Geometry: final body of the model. Coordinates: model frame, mm. A direction names the side the tool comes from. Give positions to 0.01 mm unless a question says otherwise; leave off trailing zeros. Loops run counter-clockwise (first coordinate to the right, second up) from the corner with the lowest first, then second, coordinate; pieces in that order, holes last.
from build123d import *

# Parameters (mm, degrees)
BOSS_EXTRUDE1_DEPTH      = 4.5
BOSS_EXTRUDE1_DEPTH_BACK = 4.5
SKETCH2_R                = 6.25
CUT_EXTRUDE1_DEPTH       = 2.7
CUT_EXTRUDE1_DEPTH_BACK  = 2.7
SKETCH3_R                = 2
CUT_EXTRUDE3_DEPTH       = 18
CHAMFER1_SIZE            = 2


with BuildPart() as part:
    # Sketch1 → Boss-Extrude1 (new body, two sides)
    with BuildSketch(Plane(origin=(0, 0, 0), x_dir=(0, 0, -1), z_dir=(1, 0, 0))) as boss_extrude1_sk:
        with BuildLine():
            Line((5, 8.5), (17.5, 8.5))
            Line((17.5, 8.5), (17.5, -8.5))
            Line((17.5, -8.5), (-17.5, -8.5))
            Line((-17.5, -8.5), (-17.5, 8.5))
            Line((-17.5, 8.5), (-5, 8.5))
            ThreePointArc((-5, 8.5), (0, 3.5), (5, 8.5))
        make_face()
    extrude(amount=BOSS_EXTRUDE1_DEPTH)
    extrude(boss_extrude1_sk.sketch, amount=-BOSS_EXTRUDE1_DEPTH_BACK)

    # Sketch2 → Cut-Extrude1 (cut, two sides)
    with BuildSketch(Plane(origin=(0, 0, 0), x_dir=(0, 0, -1), z_dir=(1, 0, 0))) as cut_extrude1_sk:
        with Locations((0, 8.5)):
            Circle(SKETCH2_R)
    extrude(amount=CUT_EXTRUDE1_DEPTH, mode=Mode.SUBTRACT)
    extrude(cut_extrude1_sk.sketch, amount=-CUT_EXTRUDE1_DEPTH_BACK, mode=Mode.SUBTRACT)

    # Sketch3 → Cut-Extrude3 (cut, through all)
    with BuildSketch(Plane(origin=(0, 8.5, 0), x_dir=(1, 0, 0), z_dir=(0, 1, 0))):
        with Locations((0, 12.5)):
            Circle(SKETCH3_R)
        with Locations((0, -12.5)):
            Circle(SKETCH3_R)
    extrude(amount=-CUT_EXTRUDE3_DEPTH, mode=Mode.SUBTRACT)

    # Chamfer1
    chamfer1_edges = [part.edges().sort_by_distance(p)[0] for p in [
        (0, 8.5, 17.5),
        (0, 8.5, -17.5),
    ]]
    chamfer(chamfer1_edges, length=CHAMFER1_SIZE)


solid = part.part
Item 1: Section query D-D on z = 4. Return loops of the section in (x, y), plus the area to 3 significant figures.
Values follow:
outline: (-4.5, -8.5) - (4.5, -8.5) - (4.5, 5.5) - (2.7, 5.5) - (2.7, 3.7) - (-2.7, 3.7) - (-2.7, 5.5) - (-4.5, 5.5) - close
area: 116 mm2
Item 2: Section query C-C on z = 0. Return loops of the section in (x, y), plus the area to 3 significant figures.
Values follow:
outline: (-4.5, -8.5) - (4.5, -8.5) - (4.5, 3.5) - (2.7, 3.5) - (2.7, 2.25) - (-2.7, 2.25) - (-2.7, 3.5) - (-4.5, 3.5) - close
area: 101 mm2
Item 3: Draft query along X for faces 1 (the face through (-4.5, 0, 0)), 2 (the face through (-2.7, 3, 0)), 3 (the face through (0, -1, 17.5)). Return one class per face: +X half, -X half, draft (parallel to the pull), parting line (faces both ways), or undercut.
Values follow:
face 1: -X half
face 2: undercut
face 3: draft
Item 4: Ray query, probe 1 along Z at (x, y) = (0, -1); probe 2 along X at (y, z) = (-2, -12.5); probe 3 along Z at (x, y) = (-1, 3.25). Return the intervals inside material, ascending.
Values follow:
probe 1: z = -17.5 to -14.5, -10.5 to 10.5, 14.5 to 17.5
probe 2: x = -4.5 to -2, 2 to 4.5
probe 3: z = -17.5 to -14.23, -10.77 to -3.39, 3.39 to 10.77, 14.23 to 17.5
Item 5: Set-up query: faces 4 (the face through (0, 7, 17)), 5 (the face through (2.7, 3, 0)). Return all of +Z, -Z, +X, -X, +Y, -Y with unobstructed straight access to the full face (end or side cutting, diameter ignored); none if empty.
Values follow:
face 4: +Z, +X, -X, +Y
face 5: +Y
Item 6: Section query B-B on y = -4.25. Return loops of the section in (x, z).
Values follow:
outline: (-4.5, -17.5) - (4.5, -17.5) - (4.5, 17.5) - (-4.5, 17.5) - close; hole circle Ø4 at (0, -12.5); hole circle Ø4 at (0, 12.5)
Item 7: Section query A-A on z = 12.5. Return loops of the section in (x, y), plus the area to 3 significant figures.
Values follow:
outline: (-4.5, -8.5) - (-2, -8.5) - (-2, 8.5) - (-4.5, 8.5) - close; (2, -8.5) - (4.5, -8.5) - (4.5, 8.5) - (2, 8.5) - close
area: 85.0 mm2
